Autodesk Inventor part; units mm, degrees
ref_plane "YZ Plane" through (0, 0, 0) normal (1, 0, 0) x (0, 1, 0)
ref_plane "XZ Plane" through (0, 0, 0) normal (0, 1, 0) x (-1, 0, 0)
ref_plane "XY Plane" through (0, 0, 0) normal (0, 0, 1) x (1, 0, 0)
sketch "Sketch1" plane through (0, 0, 0) normal (0, 0, 1) x (1, 0, 0)
  line L0 (-1.0667, -1.8887) -> (-0.1724, 23.0976)
  line L1 (0.8627, 24.0612) -> (4.8545, 23.9183)
  line L2 (5.8181, 22.8832) -> (4.9238, -2.1031)
  line L3 (3.8887, -3.0667) -> (-0.1031, -2.9238)
  circle A0 centre (2, 0) radius 1.4986
  circle A1 centre (2.7514, 20.9945) radius 1.4986
  circle A2 centre (2.7514, 20.9945) radius 1.4986
  circle A3 centre (2, 0) radius 1.4986
  arc A4 (-1.0667, -1.8887) -> (-0.1031, -2.9238) centre (-0.0674, -1.9245) ccw
  arc A5 (3.8887, -3.0667) -> (4.9238, -2.1031) centre (3.9245, -2.0674) ccw
  arc A6 (5.8181, 22.8832) -> (4.8545, 23.9183) centre (4.8188, 22.919) ccw
  arc A7 (0.8627, 24.0612) -> (-0.1724, 23.0976) centre (0.8269, 23.0619) ccw
  point P0 (0, 0)
  dimension "d0" = 5.9944
  dimension "d1" = 2.9972
  dimension "d2" = 2.9972
  dimension "d3" = 2.9972
  dimension "d4" = 2.9972
  dimension "d6" = 2.9972
  dimension "d7" = 2.9972
  dimension "d8" = 1
extrude "Extrusion1" add sketch "Sketch1" along normal blind 3
equation "\"d2\" = d1"
equation "\"d3\" = d2"
equation "\"d4\" = d2"
equation "\"d6\" = d1"
properties part number "Connector Boi"
The model under review builds one solid part; all positions refer to its coordinate system, in mm. Round coordinates to 2 decimals unless told otherwise and drop trailing zeros. Write each loop counter-clockwise with the first axis right and the second up, starting at its lowest first coordinate (ties: lowest second). Pieces come first, ordered by that corner, then holes.
(1) We need section A-A on x = 1.75. Give the boundary of the cut face in (y, z).
(2) We need section B-B on z = 1. Give the boundary of the cut face in (x, y).
(3) We need section C-C on y = 21.25. Give the boundary of the cut face in (x, z), and give its area (3 significant figures).
(4) Mouldability with a two-part tool opening along Y and no side actions: class faces 1 (the cylindrical face through (2.56, 19.51, 1.48)), 2 (the cylindrical face through (3.43, -0.45, 1.48)), 3 (the cylindrical face through (4.614, -2.792, 1.479)), 4 (the flat face through (2, 11, 3)) as +Y half, -Y half, draft (parallel to the pull), parting line (faces both ways), or undercut.
(5) We need section D-D on y = 0. Give the boundary of the cut face in (x, z).
(6) Wall thickness on L1, parallel to Y at x = 2, z = 2; L2, parallel to Y at x = 1, z = 1.8; L3, parallel to X at y = -0.75, z = 1.4: over which ranges is each line inside the solid? List them lowest first.
Findings below:
1. outline: (-2.99, 0) - (-1.48, 0) - (-1.48, 3) - (-2.99, 3) - close; (1.48, 0) - (19.88, 0) - (19.88, 3) - (1.48, 3) - close; (22.11, 0) - (24.03, 0) - (24.03, 3) - (22.11, 3) - close
2. outline: (-1.07, -1.89) arc R1 ccw to (-0.1, -2.92) - (3.89, -3.07) arc R1 ccw to (4.92, -2.1) - (5.82, 22.88) arc R1 ccw to (4.85, 23.92) - (0.86, 24.06) arc R1 ccw to (-0.17, 23.1) - close; hole circle Ø3 at (2, 0); hole circle Ø3 at (2.75, 20.99)
3. outline: (-0.24, 0) - (1.27, 0) - (1.27, 3) - (-0.24, 3) - close; (4.23, 0) - (5.76, 0) - (5.76, 3) - (4.23, 3) - close
3. area: 9.13 mm2
4. face 1: undercut
4. face 2: undercut
4. face 3: -Y half
4. face 4: draft
5. outline: (-1, 0) - (0.5, 0) - (0.5, 3) - (-1, 3) - close; (3.5, 0) - (5, 0) - (5, 3) - (3.5, 3) - close
6. L1: y = -3 to -1.5, 1.5 to 19.7, 22.29 to 24.02
6. L2: y = -2.96 to -1.12, 1.12 to 24.06
6. L3: x = -1.03 to 0.7, 3.3 to 4.97
